Read the model definition and answer for the solid it produces. Units are mm, in the model's axes. Face numbers are marked on the shaded views. A direction names the side the tool comes from. Coordinates: 2 decimals unless noted, no trailing zeros. Write each loop counter-clockwise with the first axis right and the second up, starting at its lowest first coordinate (ties: lowest second). Pieces come first, ordered by that corner, then holes. Notation, with made-up numbers: (79.5, -23) -> (84.5, -23) arc R25 cw to (84.5, 2) -> close; hole circle Ø3 at (27, 38.25). An arc over 180 degrees is marked (long way). One line per item, written item: value. Start each with the question number.
1. Find section C-C, the plane x = 11.75. Write down the section's boundary in (y, z).
2. For the marked faces 1, 2 and 3, determine the directions among +Z, -Z, +X, -X, +Y, -Y from which every point of the face is accessible in a straight line to the end or side of a thin tool.
3. Find section A-A, the plane y = 7. Write down the section's boundary in (x, z), and give its area (3 significant figures).
4. Given P1, Ø5, axis at x = 2.5, z = 14.5, coming from the -Y side; P2, Ø5, axis at x = 16.5, y = 3.5, coming from the +Z side; P3, Ø5, axis at y = 7.5, z = 13.5, coming from the +X side; P4, Ø3, axis at x = 6, y = 5, coming from the +Z side, each flat-ended and moving along its own axis, determine where each tip first touches the part or whether it passes through.
5. Consider line 1 along X through (y, z) = (7, 11.75); line 2 along Z through (x, y) = (4.5, 2). Determine where each line is inside the solid, lowest interval first.
6. Find section B-B, the plane z = 11. Write down the section's boundary in (x, y), and give its area (3 significant figures).
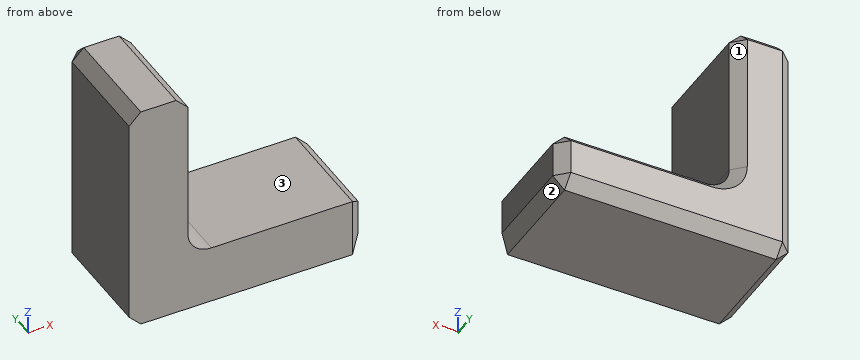
```python
from build123d import *

# Parameters (mm, degrees)
EXTRUDE_1_DEPTH = 10
FILLET_1_R      = 2
CHAMFER_1_SIZE  = 1


with BuildPart() as part:
    # 草图1 → 凸台-拉伸1 (new body)
    with BuildSketch(Plane(origin=(0, 0, 0), x_dir=(1, 0, 0), z_dir=(0, 1, 0))):
        Polygon((5, 0), (0, 0), (0, -5), (0, -20), (5, -20), (5, -5), (20, -5), (20, 0), align=None)
    extrude(amount=EXTRUDE_1_DEPTH)

    # 圆角1
    fillet_1_edges = [part.edges().sort_by_distance(p)[0] for p in [
        (5, 5, 5),
    ]]
    fillet(fillet_1_edges, radius=FILLET_1_R)

    # 倒角1
    chamfer_1_edges = [part.edges().sort_by_distance(p)[0] for p in [
        (20, 0, 2.5),
        (10, 10, 0),
        (20, 5, 5),
        (5, 5, 20),
        (0, 5, 20),
        (0, 5, 0),
        (20, 5, 0),
        (0, 10, 10),
        (2.5, 10, 20),
        (13.5, 10, 5),
        (5, 10, 13.5),
        (5.585786438, 10, 5.585786438),
        (20, 10, 2.5),
    ]]
    chamfer(chamfer_1_edges, length=CHAMFER_1_SIZE)


solid = part.part
```
Answer block:
1. outline: (0, 0) -> (9, 0) -> (10, 1) -> (10, 4) -> (9, 5) -> (0, 5) -> close
2. face 1: +Z, +X, +Y
2. face 2: -Z, +X, +Y, -Y
2. face 3: +Z, +X, +Y, -Y
3. outline: (0, 1) -> (1, 0) -> (19, 0) -> (20, 1) -> (20, 4) -> (19, 5) -> (7, 5) arc R2 cw to (5, 7) -> (5, 19) -> (4, 20) -> (1, 20) -> (0, 19) -> close
3. area: 173 mm2
4. P1: stops at y = 0
4. P2: stops at z = 5
4. P3: stops at x = 5
4. P4: stops at z = 19.5
5. line 1: x = 0 to 5
5. line 2: z = 0 to 19.5
6. outline: (0, 0) -> (5, 0) -> (5, 9) -> (4, 10) -> (1, 10) -> (0, 9) -> close
6. area: 49.0 mm2
